The listing builds one solid part. Answer for the finished solid, in the listing's coordinates (mm). Coordinates: 2 decimals unless noted, no trailing zeros. Order: outer loops, then holes, each group sorted by start corner. A loop starts at its lowest first (then second) coordinate and runs counter-clockwise, first axis right, second up. Notation, with made-up numbers: (-23, 53) - (15, 53) arc R26 cw to (15, 69) - close; hole circle Ø10 at (52.5, 16). An arc over 180 degrees is marked (long way). One line per item, written item: value. Start each with the question number.
Autodesk Inventor part; units mm, degrees
ref_plane "YZ Plane" through (0, 0, 0) normal (1, 0, 0) x (0, 1, 0)
ref_plane "XZ Plane" through (0, 0, 0) normal (0, 1, 0) x (-1, 0, 0)
ref_plane "XY Plane" through (0, 0, 0) normal (0, 0, 1) x (1, 0, 0)
sketch "Sketch1" plane through (0, 0, 0) normal (1, 0, 0) x (0, 1, 0)
  line L0 (4.3974, 6.5718) -> (-1.9526, 6.5718)
  line L1 (-1.9526, 6.5718) -> (-1.9526, -12.4782)
  line L2 (-1.9526, -12.4782) -> (4.3974, -12.4782)
  line L3 (4.3974, -12.4782) -> (4.3974, 6.5718)
  point P0 (0, 0)
  dimension "d0" = 19.05
  dimension "d1" = 6.35
extrude "Extrusion1" add sketch "Sketch1" along normal blind 1.5875
sketch "Sketch2" plane through (1.5875, 0, 0) normal (1, 0, 0) x (0, 0, -1)
  line L0 (12.4782, 4.3974) -> (-6.5718, 4.3974)
  line L1 (-6.5718, 4.3974) -> (-6.5718, -1.9526)
  line L2 (12.4782, -1.9526) -> (12.4782, 4.3974)
  point P0 (0, 0)
  point P1 (-3.3968, 1.2224)
  point P2 (9.3032, 1.2224)
  dimension "d4" = 3.175
  dimension "d5" = 3.175
  dimension "d6" = 3.175
hole "Hole1" at (1.5875, 1.2224, 3.3968) at (1.5875, 1.2224, -9.3032) direction (-1, 0, 0) diameter 3.302 depth 25.4 tip angle 118.188
properties part number "clampPlate"
(1) Consider probe 1 along Z at (x, y) = (1.2, 1); probe 2 along Z at (x, y) = (0.6, 0.25); probe 3 along Y at (x, z) = (1.1, 3.5). Determine where each line is inside the solid, lowest interval first.
(2) The part is cut by section B-B on z = 4.5. Determine the outline of the cut face in (x, y), plus the area to 3 significant figures.
(3) The part is cut by section C-C on x = 0.6. Determine the outline of the cut face in (y, z).
(4) For a pull along Z with two mould halves and no side action, classify faces 1 (the face through (1.588, 1, -3)), 2 (the face through (1, 1, -12.478)), 3 (the face through (0.78, 0.73, -10.88)) as pulls with the +Z half, pulls with the -Z half, needs draft (parallel to the pull), parting line crosses it, or undercut.
(5) The part is cut by section D-D on z = -8. Determine the outline of the cut face in (x, y).
(6) The part is cut by section A-A on y = 1.75. Determine the outline of the cut face in (x, z), plus the area to 3 significant figures.
Completed:
1. probe 1: z = -12.48 to -10.94, -7.67 to 1.76, 5.03 to 6.57
1. probe 2: z = -12.48 to -10.64, -7.97 to 2.06, 4.73 to 6.57
1. probe 3: y = -1.95 to -0.43, 2.87 to 4.4
2. outline: (0, -1.95) - (1.59, -1.95) - (1.59, -0.01) - (0, -0.01) - close; (0, 2.45) - (1.59, 2.45) - (1.59, 4.4) - (0, 4.4) - close
2. area: 6.18 mm2
3. outline: (-1.95, -12.48) - (4.4, -12.48) - (4.4, 6.57) - (-1.95, 6.57) - close; hole circle Ø3.3 at (1.22, -9.3); hole circle Ø3.3 at (1.22, 3.4)
4. face 1: needs draft
4. face 2: pulls with the -Z half
4. face 3: undercut
5. outline: (0, -1.95) - (1.59, -1.95) - (1.59, 0.21) - (0, 0.21) - close; (0, 2.24) - (1.59, 2.24) - (1.59, 4.4) - (0, 4.4) - close
6. outline: (0, -12.48) - (1.59, -12.48) - (1.59, -10.87) - (0, -10.87) - close; (0, -7.74) - (1.59, -7.74) - (1.59, 1.83) - (0, 1.83) - close; (0, 4.96) - (1.59, 4.96) - (1.59, 6.57) - (0, 6.57) - close
6. area: 20.3 mm2
